Input: part model. Units: mm. Frame: model coordinates. Face numbers are marked on the shaded views. A direction names the side the tool comes from. Coordinates: 2 decimals unless noted, no trailing zeros. Loops run counter-clockwise (first coordinate to the right, second up) from the corner with the lowest first, then second, coordinate; pieces in that order, holes last.
Item 1: Reachability of the marked faces 1, 2 and 3 from +Z, -Z, +X, -X, +Y, -Y: full face, straight path, thin tool, end or side. Return the list, or none.
Item 2: Contact query for flat-ended pins moving along their axis: P1, Ø1, axis at x = 18.5, y = 10.5, coming from the -Z side; P2, Ø12, axis at x = 26, y = -5, coming from the -Z side; P3, Ø9, axis at x = 8.5, z = -3, coming from the -Y side. Output: stop coordinate, or through.
Item 3: Section A-A on z = 53.5. Return loops of the section in (x, y) (3 decimals).
Item 4: Section B-B on x = 5. Return loops of the section in (y, z), and give its area (3 significant figures).
Item 5: Section C-C on y = 2.5. Return loops of the section in (x, z).
Item 6: Ray query, line 1 along Y through (x, z) = (35, 2.5) (3 decimals); line 2 along Z through (x, y) = (5, -0.25); line 3 along X through (y, z) = (-3.75, -9). Return the intervals inside material, ascending.
Item 7: Section D-D on z = -10. Return loops of the section in (x, y).
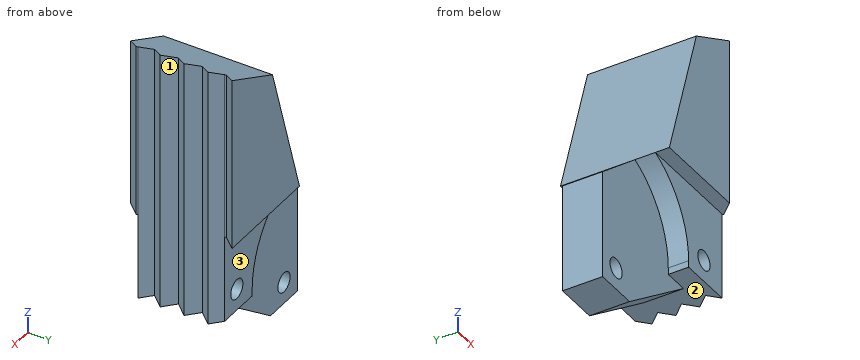
```python
from build123d import *

# Parameters (mm, degrees)
BOSS_EXTRUDE1_DEPTH  = 12.5
SKETCH3_W            = 37
SKETCH3_H            = 20
CUT_EXTRUDE1_DEPTH   = 7.9
SKETCH4_W            = 37
SKETCH4_H            = 20
CUT_EXTRUDE2_DEPTH   = 7.9
SKETCH5_W            = 20
SKETCH5_H            = 18.55
BOSS_EXTRUDE2_DEPTH  = 12.675
BOSS_EXTRUDE3_DEPTH  = 9.2
M4_CLEARANCE_HOLE1_D = 4.5
CUT_EXTRUDE3_DEPTH   = 72.590851371
FILLET1_R            = 20


with BuildPart() as part:
    # Sketch2 → Boss-Extrude1 (new, symmetric)
    with BuildSketch(Plane(origin=(0, 0, 0), x_dir=(1, 0, 0), z_dir=(0, 1, 0))):
        Polygon((0, 0), (37, 0), (37, -60), (22, -52.5), (12, -20), (0, -10), align=None)
    extrude(amount=BOSS_EXTRUDE1_DEPTH, both=True)

    # Sketch3 → Cut-Extrude1 (cut)
    with BuildSketch(Plane(origin=(0, 12.5, 0), x_dir=(1, 0, 0), z_dir=(0, 1, 0))):
        with Locations((18.5, -10)):
            Rectangle(SKETCH3_W, SKETCH3_H)
    extrude(amount=-CUT_EXTRUDE1_DEPTH, mode=Mode.SUBTRACT)

    # Sketch4 → Cut-Extrude2 (cut)
    with BuildSketch(Plane(origin=(0, -12.5, 0), x_dir=(-1, 0, 0), z_dir=(0, -1, 0))):
        with Locations((-18.5, -10)):
            Rectangle(SKETCH4_W, SKETCH4_H)
    extrude(amount=-CUT_EXTRUDE2_DEPTH, mode=Mode.SUBTRACT)

    # Sketch5 → Boss-Extrude2 (add)
    with BuildSketch(Plane(origin=(37, 0, 0), x_dir=(0, 0, -1), z_dir=(1, 0, 0))):
        with Locations((-10, 0)):
            Rectangle(SKETCH5_W, SKETCH5_H)
    extrude(amount=-BOSS_EXTRUDE2_DEPTH)

    # Sketch10 → Boss-Extrude3 (add)
    with BuildSketch(Plane(origin=(0, 4.6, 0), x_dir=(1, 0, 0), z_dir=(0, 1, 0))):
        Polygon((30, 0), (10, 15), (0, 15), (0, 0), align=None)
    extrude(amount=-BOSS_EXTRUDE3_DEPTH)

    # M4 Clearance Hole1 (through all)
    with Locations(Plane(origin=(0, 9.275, 0), x_dir=(1, 0, 0), z_dir=(0, 1, 0))):
        with Locations((30, -5), (5, 10)):
            Hole(M4_CLEARANCE_HOLE1_D / 2)

    # Sketch8 → Cut-Extrude3 (cut, through all)
    with BuildSketch(Plane(origin=(0, 0, 0), x_dir=(-1, 0, 0), z_dir=(0, 0, -1))):
        Polygon((-34.261387212, 4), (-37, 7), (-37, 1.5), align=None)
        Polygon((-34.261387212, -1.5), (-37, 1.5), (-37, -4), align=None)
        Polygon((-34.261387212, 9.5), (-37, 12.5), (-37, 9.275), (-34.507862363, 9.275), align=None)
        Polygon((-34.507862363, 9.275), (-37, 9.275), (-37, 7), align=None)
        Polygon((-34.261387212, -7), (-37, -4), (-37, -9.275), (-36.753524849, -9.275), align=None)
        Polygon((-36.753524849, -9.275), (-37, -9.275), (-37, -9.5), align=None)
        Polygon((-34.261387212, -12.5), (-37, -9.5), (-37, -12.5), align=None)
    extrude(amount=-CUT_EXTRUDE3_DEPTH, mode=Mode.SUBTRACT)

    # Fillet1
    # the kernel refuses this fillet: 20 mm, written as the material it adds along each edge
    with BuildSketch(Plane(origin=(24.325, 41.571851206, 20), x_dir=(0, 0, -1), z_dir=(0, -1, 0))) as fillet1_piece_1_section:
        with BuildLine():
            CenterArc((18.468740482, -20), FILLET1_R, 90, 67.433839366)
            Line((0, -12.325), (-0.36937481, -12.1715))
            ThreePointArc((-0.36937481, -12.1715), (-0.4, -6.1625), (-0.4, 0))
            Line((-0.4, 0), (0, 0.4))
            Line((0, 0.4), (18.468740482, 0.4))
            Line((18.468740482, 0.4), (18.468740482, 0))
        make_face()
    fillet1_piece_1 = extrude(amount=50.846851206, mode=Mode.PRIVATE)
    fillet1_piece_1 = split(fillet1_piece_1, bisect_by=Plane(origin=(21.141865588, 9.275, 15.519731965), z_dir=(0, -1, 0)), keep=Keep.TOP, mode=Mode.PRIVATE)
    add(fillet1_piece_1)
    with BuildSketch(Plane(origin=(24.325, 9.275, 20), x_dir=(0, 0, -1), z_dir=(0, -1, 0))) as fillet1_piece_2_section:
        with BuildLine():
            CenterArc((18.468740482, -20), FILLET1_R, 90, 67.433839366)
            Line((0, -12.325), (-0.36937481, -12.1715))
            ThreePointArc((-0.36937481, -12.1715), (-0.4, -6.1625), (-0.4, 0))
            Line((-0.4, 0), (0, 0.4))
            Line((0, 0.4), (18.468740482, 0.4))
            Line((18.468740482, 0.4), (18.468740482, 0))
        make_face()
    fillet1_piece_2 = extrude(amount=50.846851206, mode=Mode.PRIVATE)
    fillet1_piece_2 = split(fillet1_piece_2, bisect_by=Plane(origin=(21.141865588, -9.275, 15.519731965), z_dir=(0, 1, 0)), keep=Keep.TOP, mode=Mode.PRIVATE)
    add(fillet1_piece_2)


solid = part.part
```
Results found:
1. face 1: +Z, -Z, +X
1. face 2: -Z, +X
1. face 3: -Z, +X, -X, +Y
2. P1: stops at z = 20
2. P2: stops at z = -7.49
2. P3: stops at y = -4.6
3. outline: (24, -12.5) - (34.261, -12.5) - (37, -9.5) - (34.261, -7) - (37, -4) - (34.261, -1.5) - (37, 1.5) - (34.261, 4) - (37, 7) - (34.261, 9.5) - (37, 12.5) - (24, 12.5) - close
4. outline: (-4.6, -15) - (4.6, -15) - (4.6, -12.25) - (-4.6, -12.25) - close; (-4.6, -7.75) - (4.6, -7.75) - (4.6, 14.17) - (-4.6, 14.17) - close
4. area: 227 mm2
5. outline: (0, -15) - (10, -15) - (30, 0) - (35.9, 0) - (35.9, 59.45) - (22, 52.5) - (12, 20) - (0, 10) - close; hole circle Ø4.5 at (5, -10); hole circle Ø4.5 at (30, 5)
6. line 1: y = -9.275 to -7.674, -6.191 to -2.174, -0.691 to 3.326, 4.809 to 8.826
6. line 2: z = -15 to -12.25, -7.75 to 14.17
6. line 3: x = 0 to 2.98, 7.02 to 18
7. outline: (0, -4.6) - (2.75, -4.6) - (2.75, 4.6) - (0, 4.6) - close; (7.25, -4.6) - (16.67, -4.6) - (16.67, 4.6) - (7.25, 4.6) - close
